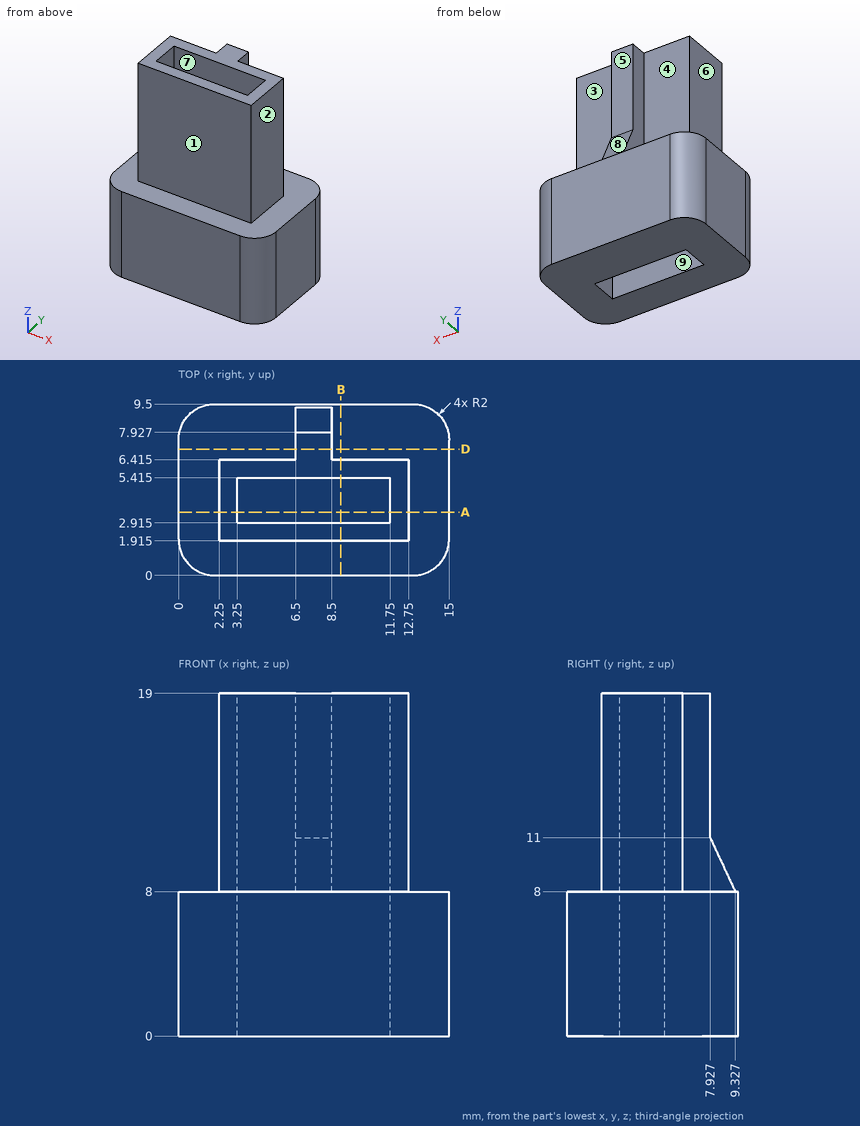
For this review, use the dimensioned drawing (mm, ordinates from the lowest corner) and the shaded views. A direction names the side the tool comes from. Give positions to 0.01 mm unless a question says otherwise; leave off trailing zeros. Order: outer loops, then holes, each group sorted by start corner. A loop starts at its lowest first (then second) coordinate and runs counter-clockwise, first axis right, second up.
1) For the marked faces 1, 2, 3, 4 and 5, list the 3-axis set-ups (+Z, -Z, +X, -X, +Y, -Y) from which the entire face can be reached by the end or side of a thin tool; tool diameter is ignored.
2) Take a section at D-D (y = 7). Give the boundary of the cut face in (x, z).
3) Insertion check: pin 1 (1 mm diameter, centred on x = 7, z = 14.5, fed in from +Y); pin 2 (2 mm diameter, centred on y = 5, z = 14, fed in from -X); pin 3 (2 mm diameter, centred on x = 4, z = 14, fed in from +Y) (1 decimal); pin 4 (2 mm diameter, centred on x = 9.5, y = 4, fed in from +Z). Each pin has a flat end and moves straight along its axis. Give the tip position at first contact, or say it passes through.
4) Wall thickness on line 1 (Y direction, x = 9, z = 16.75) (1 decimal); line 2 (Y direction, x = 7.75, z = 2.75) (1 decimal); line 3 (X direction, y = 5, z = 17.75): over which ranges is each line inside the solid? List them lowest first.
5) Take a section at A-A (y = 3.5). Give the boundary of the cut face in (x, z).
6) The part is to be moulded in two halves that separate along X. For the marked faces 6, 7, 8 and 9, say which applies: released by +X, released by -X, zero draft, split by the parting line, or undercut.
7) Take a section at B-B (x = 9). Give the boundary of the cut face in (y, z) (1 decimal), then the cut area to 3 significant figures.
Derived:
1. face 1: +Z, +X, -X, -Y
1. face 2: +Z, +X, +Y, -Y
1. face 3: +Z, +X, +Y
1. face 4: +Z, -X, +Y
1. face 5: +Z, +X, -X, +Y
2. outline: (0, 0) - (15, 0) - (15, 8) - (8.5, 8) - (8.5, 19) - (6.5, 19) - (6.5, 8) - (0, 8) - close
3. pin 1: stops at y = 7.93
3. pin 2: stops at x = 2.25
3. pin 3: stops at y = 6.4
3. pin 4: passes through
4. line 1: y = 1.9 to 2.9, 5.4 to 6.4
4. line 2: y = 0 to 2.9, 5.4 to 9.5
4. line 3: x = 2.25 to 3.25, 11.75 to 12.75
5. outline: (0, 0) - (3.25, 0) - (3.25, 19) - (2.25, 19) - (2.25, 8) - (0, 8) - close; (11.75, 0) - (15, 0) - (15, 8) - (12.75, 8) - (12.75, 19) - (11.75, 19) - close
6. face 6: released by -X
6. face 7: undercut
6. face 8: zero draft
6. face 9: undercut
7. outline: (0, 0) - (2.9, 0) - (2.9, 19) - (1.9, 19) - (1.9, 8) - (0, 8) - close; (5.4, 0) - (9.5, 0) - (9.5, 8) - (6.4, 8) - (6.4, 19) - (5.4, 19) - close
7. area: 78.0 mm2
